```python
from build123d import *

# Parameters (mm, degrees)
F0_W     = 102.489
F0_H     = 102.489
F1_DEPTH = 3.175
F2_W     = 50.8
F2_H     = 44.45
F3_DEPTH = 3.175
F4_R     = 6.3246
F5_R     = 4.7625
F7_DEPTH = 3.175
F9_DEPTH = 47.625
F9_TAPER = 1
F10_R    = 3.175


with BuildPart() as f1:
    # F0 (on Top) → F1 (new body)
    with BuildSketch(Plane.XY):
        Rectangle(F0_W, F0_H)
    extrude(amount=F1_DEPTH)

    # F2 (on face) → F3 (join)
    with BuildSketch(Plane.XY.offset(3.175)):
        with Locations((0, -73.4695)):
            Rectangle(F2_W, F2_H)
    extrude(amount=-F3_DEPTH)

    # F4
    f4_edges = [f1.edges().sort_by_distance(p)[0] for p in [
        (25.4, -95.6945, 1.5875),
        (-25.4, -95.6945, 1.5875),
    ]]
    fillet(f4_edges, radius=F4_R)

    # F5
    f5_edges = [f1.edges().sort_by_distance(p)[0] for p in [
        (-51.2445, -51.2445, 1.5875),
        (51.2445, -51.2445, 1.5875),
        (51.2445, 51.2445, 1.5875),
        (-51.2445, 51.2445, 1.5875),
    ]]
    fillet(f5_edges, radius=F5_R)

    # F6 (on face) → F7 (join)
    with BuildSketch(Plane.XY.offset(3.175)):
        with BuildLine():
            Line((-25.4, 11.049), (-25.4, -47.6885))
            Line((-25.4, -47.6885), (-23.0632, -47.6885))
            Line((-23.0632, -47.6885), (-23.0632, 10.2997))
            ThreePointArc((-23.0632, 10.2997), (-22.5982320151, 11.4222320151), (-21.4757, 11.8872))
            Line((-21.4757, 11.8872), (21.4757, 11.8872))
            ThreePointArc((21.4757, 11.8872), (22.5982320151, 11.4222320151), (23.0632, 10.2997))
            Line((23.0632, 10.2997), (23.0632, -47.6885))
            Line((23.0632, -47.6885), (25.4, -47.6885))
            Line((25.4, -47.6885), (25.4, 11.049))
            ThreePointArc((25.4, 11.049), (24.4700640303, 13.2940640303), (22.225, 14.224))
            Line((22.225, 14.224), (-22.225, 14.224))
            ThreePointArc((-22.225, 14.224), (-24.4700640303, 13.2940640303), (-25.4, 11.049))
        make_face()
        with BuildLine():
            Line((25.4, -89.3699), (25.4, -51.2445))
            Line((25.4, -51.2445), (23.0632, -51.2445))
            Line((23.0632, -51.2445), (23.0632, -89.3699))
            ThreePointArc((23.0632, -89.3699), (21.895200422, -92.189700422), (19.0754, -93.3577))
            Line((19.0754, -93.3577), (-19.0754, -93.3577))
            ThreePointArc((-19.0754, -93.3577), (-21.895200422, -92.189700422), (-23.0632, -89.3699))
            Line((-23.0632, -89.3699), (-23.0632, -51.2445))
            Line((-23.0632, -51.2445), (-25.4, -51.2445))
            Line((-25.4, -51.2445), (-25.4, -89.3699))
            ThreePointArc((-25.4, -89.3699), (-23.5475675483, -93.8420675483), (-19.0754, -95.6945))
            Line((-19.0754, -95.6945), (19.0754, -95.6945))
            ThreePointArc((19.0754, -95.6945), (23.5475675483, -93.8420675483), (25.4, -89.3699))
        make_face()
    extrude(amount=F7_DEPTH)

    # F8 (on face) → F9 (join)
    with BuildSketch(Plane.XY.offset(6.35)):
        with BuildLine():
            Line((-21.4757, 11.8872), (21.4757, 11.8872))
            ThreePointArc((21.4757, 11.8872), (22.5982320151, 11.4222320151), (23.0632, 10.2997))
            Line((23.0632, 10.2997), (23.0632, -4.826))
            Line((23.0632, -4.826), (25.4, -4.826))
            Line((25.4, -4.826), (25.4, 11.049))
            ThreePointArc((25.4, 11.049), (24.4700640303, 13.2940640303), (22.225, 14.224))
            Line((22.225, 14.224), (-22.225, 14.224))
            ThreePointArc((-22.225, 14.224), (-24.4700640303, 13.2940640303), (-25.4, 11.049))
            Line((-25.4, 11.049), (-25.4, -4.826))
            Line((-25.4, -4.826), (-23.0632, -4.826))
            Line((-23.0632, -4.826), (-23.0632, 10.2997))
            ThreePointArc((-23.0632, 10.2997), (-22.5982320151, 11.4222320151), (-21.4757, 11.8872))
        make_face()
    extrude(amount=F9_DEPTH, taper=F9_TAPER)

    # F10
    f10_edges = [f1.edges().sort_by_distance(p)[0] for p in [
        (-24.2316, -3.994703, 53.975),
        (24.2316, -3.994703, 53.975),
    ]]
    fillet(f10_edges, radius=F10_R)


solid = f1.part
```
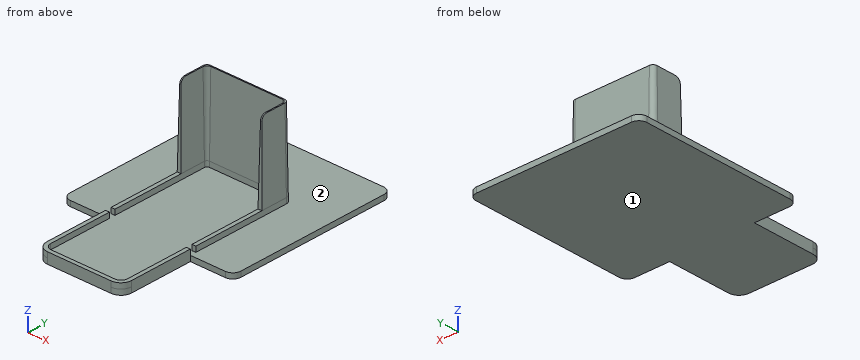
Could you check a few things on this model? Use its own coordinates, in mm. Face numbers are marked on the shaded views. Round coordinates to 2 decimals unless told otherwise and drop trailing zeros. Loops run counter-clockwise (first coordinate to the right, second up) from the corner with the lowest first, then second, coordinate; pieces in that order, holes last. Notation, with made-up numbers: M 33,18 L 75,18 A33 ccw 75,47 Z; hole C 66,73.25 d7. An arc over 180 degrees is marked long. Answer as CSV lines item,"result".
1) Imagine slicing it at A-A on y = -56.5. List the corners of the cut face in (x, z) for me (3 decimals).
From the geometry:
outline,"M -25.4,0 L 25.4,0 L 25.4,6.35 L 23.063,6.35 L 23.063,3.175 L -23.063,3.175 L -23.063,6.35 L -25.4,6.35 Z"
2) We'd pull the mould along Y, two halves only. Please class the marked faces 1 and 2: released by +Y, released by -Y, zero draft, split by the parting line, or undercut.
From the geometry:
face 1,"zero draft"
face 2,"undercut"
3) Imagine slicing it at D-D on y = 23. List the corners of the cut face in (x, z) for me (1 decimal).
From the geometry:
outline,"M -51.2,0 L 51.2,0 L 51.2,3.2 L -51.2,3.2 Z"
4) For pin 1 Ø3.5 at (y, z) = (-70.5, 5) entering from -X; pin 2 Ø3.5 at (y, z) = (-79, 5.5) entering from +X; pin 3 Ø5 at (x, z) = (-8.5, 31.5) entering from -Y; pin 4 Ø5 at (x, z) = (28, 36.5) entering from +Y, each with a flat end and sliding along its axis, tell me the tip position at first contact or that it passes through.
From the geometry:
pin 1,"x = -25.4"
pin 2,"x = 25.4"
pin 3,"y = 12.28"
pin 4,"through"
5) Imagine slicing it at C-C on z = 20.5. List the corners of the cut face in (x, y) for me (3 decimals), and give its area (3 significant figures).
From the geometry:
outline,"M -25.153,-4.579 L -23.31,-4.579 L -23.31,10.3 A1.834 cw -21.476,12.134 L 21.476,12.134 A1.834 cw 23.31,10.3 L 23.31,-4.579 L 25.153,-4.579 L 25.153,11.049 A2.928 ccw 22.225,13.977 L -22.225,13.977 A2.928 ccw -25.153,11.049 Z"
area,"152 mm^2"
6) If I drill on probe 1 along Z at (x, y) = (15, -69) (3 decimals); probe 2 along X at (y, z) = (3, 21); probe 3 along X at (y, z) = (-2, 40), over which ranges is the centre line in solid material (lowest first)?
From the geometry:
probe 1,"0 to 3.175"
probe 2,"-25.14 to -23.32, 23.32 to 25.14"
probe 3,"-24.81 to -23.65, 23.65 to 24.81"
